from build123d import *

# Parameters (mm, degrees)
BODYSKE_R   = 0.6
BODY_DEPTH  = 0.7
NOTSKE_W    = 1.9
NOTSKE_H    = 1.2
NOTCH_DEPTH = 7.733295861


with BuildPart() as part:
    # BodySke → Body (new body)
    with BuildSketch(Plane.XY):
        with BuildLine():
            Line((0.089864865, -2.848582859), (0.175, -5.547240305))
            ThreePointArc((0.175, -5.547240305), (0.943397685, -5.469232195), (1.693525559, -5.285307104))
            ThreePointArc((1.693525559, -5.285307104), (2.040324005, -5.051829297), (2.2082544, -4.668971058))
            Line((2.2082544, -4.668971058), (2.421252601, -3.051089095))
            ThreePointArc((2.421252601, -3.051089095), (2.576047275, -2.4964236), (2.879326572, -2.006896409))
            ThreePointArc((2.879326572, -2.006896409), (0, 4.15), (-2.879326572, -2.006896409))
            ThreePointArc((-2.879326572, -2.006896409), (-2.576047275, -2.4964236), (-2.421252601, -3.051089095))
            Line((-2.421252601, -3.051089095), (-2.2082544, -4.668971058))
            ThreePointArc((-2.2082544, -4.668971058), (-2.040324005, -5.051829297), (-1.693525559, -5.285307104))
            ThreePointArc((-1.693525559, -5.285307104), (-0.943397685, -5.469232195), (-0.175, -5.547240305))
            Line((-0.175, -5.547240305), (-0.089864865, -2.848582859))
            ThreePointArc((-0.089864865, -2.848582859), (0, 2.85), (0.089864865, -2.848582859))
        make_face()
        with Locations((0.95, -4.168108084)):
            Circle(BODYSKE_R, mode=Mode.SUBTRACT)
        with Locations((-0.95, -4.168108084)):
            Circle(BODYSKE_R, mode=Mode.SUBTRACT)
    extrude(amount=-BODY_DEPTH)

    # NotSke → Notch (cut, through all)
    with BuildSketch(Plane.XY):
        with Locations((0, -4.168108084)):
            Rectangle(NOTSKE_W, NOTSKE_H)
    extrude(amount=-NOTCH_DEPTH, mode=Mode.SUBTRACT)


solid = part.part
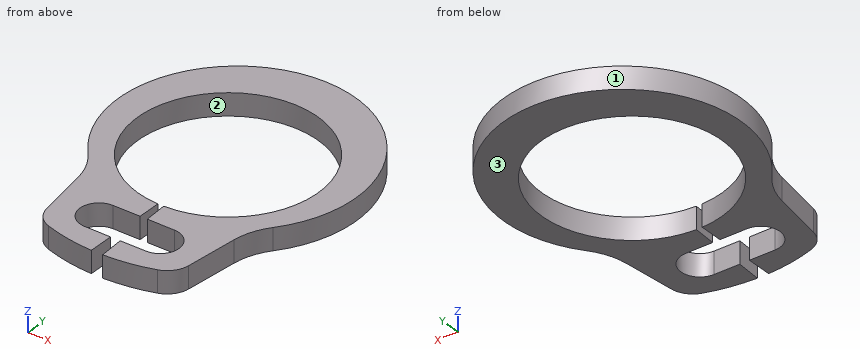
Design review of the part built by this model. Coordinates are the model's own, in mm. Face numbers are marked on the shaded views. Coordinates: 2 decimals unless noted, no trailing zeros. Order: outer loops, then holes, each group sorted by start corner. A loop starts at its lowest first (then second) coordinate and runs counter-clockwise, first axis right, second up. Notation, with made-up numbers: (-32.5, 65) -> (-16.5, 65) arc R16 ccw to (-16.5, 95) -> close; hole circle Ø1 at (82.5, -12.5). An arc over 180 degrees is marked (long way). One line per item, written item: value.
1) We need section B-B, the plane z = -0.1. Give the boundary of the cut face in (x, y) (3 decimals).
Output values:
outline: (-2.879, -2.007) arc R2.045 cw to (-2.421, -3.051) -> (-2.208, -4.669) arc R0.75 ccw to (-1.694, -5.285) arc R5.55 ccw to (-0.175, -5.547) -> (-0.15, -4.768) -> (-0.95, -4.768) arc R0.6 cw to (-0.95, -3.568) -> (-0.113, -3.568) -> (-0.09, -2.849) arc R2.85 cw (long way) to (0.09, -2.849) -> (0.113, -3.568) -> (0.95, -3.568) arc R0.6 cw to (0.95, -4.768) -> (0.15, -4.768) -> (0.175, -5.547) arc R5.55 ccw to (1.694, -5.285) arc R0.75 ccw to (2.208, -4.669) -> (2.421, -3.051) arc R2.045 cw to (2.879, -2.007) arc R3.752 ccw (long way) to start
2) We need section D-D, the plane y = 3.5. Give the boundary of the cut face in (x, z).
Output values:
outline: (-2.11, -0.7) -> (2.11, -0.7) -> (2.11, 0) -> (-2.11, 0) -> close
3) To check wall thickness, follow probe 1 along Y at (x, z) = (-1, -0.55); probe 2 along Y at (x, z) = (-0.25, -0.6); probe 3 along X at (y, z) = (1.5, -0.2). State the ranges of each line that lie inside material, in increasing order. Write a range as [from, to].
Output values:
probe 1: y = [-5.46, -4.77], [-3.57, -2.67], [2.67, 4.01]
probe 2: y = [-5.54, -4.77], [-3.57, -2.84], [2.84, 4.14]
probe 3: x = [-3.59, -2.42], [2.42, 3.59]
4) Draft analysis for pull direction Y (two halves, no side actions). For the marked faces 1, 2 and 3, state which applies: +Y half, -Y half, draft (parallel to the pull), parting line (faces both ways), or undercut.
Output values:
face 1: parting line
face 2: undercut
face 3: draft
5) We need section A-A, the plane y = 0.75. Give the boundary of the cut face in (x, z).
Output values:
outline: (-3.74, -0.7) -> (-2.75, -0.7) -> (-2.75, 0) -> (-3.74, 0) -> close; (2.75, -0.7) -> (3.74, -0.7) -> (3.74, 0) -> (2.75, 0) -> close
6) We need section C-C, the plane x = -2. Give the boundary of the cut face in (y, z), then the cut area to 3 significant figures.
Output values:
outline: (-5.1, -0.7) -> (-2.03, -0.7) -> (-2.03, 0) -> (-5.1, 0) -> close; (2.03, -0.7) -> (3.57, -0.7) -> (3.57, 0) -> (2.03, 0) -> close
area: 3.23 mm2
